from build123d import *

# Parameters (mm, degrees)
SKETCH1_W               = 138
SKETCH1_H               = 63
BOSS_EXTRUDE1_DEPTH     = 2.5
SKETCH3_W               = 28
SKETCH3_H               = 6
CUT_EXTRUDE2_DEPTH      = 10
SKETCH4_W               = 61
SKETCH4_H               = 22
CUT_EXTRUDE3_DEPTH      = 2
SKETCH6_W               = 33
SKETCH6_H               = 19
CUT_EXTRUDE5_DEPTH      = 1.5
SKETCH11_R              = 0.775
CUT_EXTRUDE8_DEPTH      = 6
CUT_EXTRUDE9_DEPTH      = 82.077123777
CUT_EXTRUDE9_DEPTH_BACK = 82.077123777
SKETCH5_R               = 1.575
SKETCH5_R_2             = 1.75
SKETCH16_R              = 6
CUT_EXTRUDE10_DEPTH     = 11
SKETCH19_R              = 1.25
CUT_EXTRUDE12_DEPTH     = 5
SKETCH21_W              = 17
SKETCH21_H              = 2.5
BOSS_EXTRUDE2_DEPTH     = 11
SKETCH22_W              = 63
SKETCH22_H              = 5
BOSS_EXTRUDE3_DEPTH     = 4
SKETCH23_R              = 1.5
BOSS_EXTRUDE4_DEPTH     = 2
FILLET3_R               = 4
FILLET2_R               = 1.5


with BuildPart() as part:
    # Sketch1 → Boss-Extrude1 (new, symmetric)
    with BuildSketch(Plane(origin=(0, 0, 0), x_dir=(1, 0, 0), z_dir=(0, 1, 0))):
        Rectangle(SKETCH1_W, SKETCH1_H)
    extrude(amount=BOSS_EXTRUDE1_DEPTH, both=True)

    # Sketch3 → Cut-Extrude2 (cut)
    with BuildSketch(Plane(origin=(0, 2.5, 0), x_dir=(1, 0, 0), z_dir=(0, 1, 0))):
        with Locations((-36, -14)):
            Rectangle(SKETCH3_W, SKETCH3_H)
        with Locations((36, -14)):
            Rectangle(SKETCH3_W, SKETCH3_H)
        with Locations((36, 14)):
            Rectangle(SKETCH3_W, SKETCH3_H)
        with Locations((-36, 14)):
            Rectangle(SKETCH3_W, SKETCH3_H)
    extrude(amount=-CUT_EXTRUDE2_DEPTH, mode=Mode.SUBTRACT)

    # Sketch4 → Cut-Extrude3 (cut)
    with BuildSketch(Plane(origin=(0, 2.5, 0), x_dir=(1, 0, 0), z_dir=(0, 1, 0))):
        with Locations((-2.5, 0)):
            Rectangle(SKETCH4_W, SKETCH4_H)
    extrude(amount=-CUT_EXTRUDE3_DEPTH, mode=Mode.SUBTRACT)

    # Sketch6 → Cut-Extrude5 (cut)
    with BuildSketch(Plane(origin=(0, 0.5, 0), x_dir=(1, 0, 0), z_dir=(0, 1, 0))):
        with Locations((7.5, 0)):
            Rectangle(SKETCH6_W, SKETCH6_H)
    extrude(amount=-CUT_EXTRUDE5_DEPTH, mode=Mode.SUBTRACT)

    # Sketch11 → Cut-Extrude8 (cut)
    with BuildSketch(Plane(origin=(0, 2.5, 0), x_dir=(1, 0, 0), z_dir=(0, 1, 0))):
        with Locations(Location((-58, 7.62, 0), (0, 0, 270))):
            Circle(SKETCH11_R)
        with Locations(Location((-19.9, 7.62, 0), (0, 0, 270))):
            Circle(SKETCH11_R)
        with Locations(Location((-58, -7.62, 0), (0, 0, 270))):
            Circle(SKETCH11_R)
        with Locations(Location((-19.9, -7.62, 0), (0, 0, 270))):
            Circle(SKETCH11_R)
    extrude(amount=-CUT_EXTRUDE8_DEPTH, mode=Mode.SUBTRACT)

    # Sketch5 → Cut-Extrude9 (cut, two sides: drawn at the far end of the back side and taken through both)
    with BuildSketch(Plane(origin=(0, 0, -11), x_dir=(-1, 0, 0), z_dir=(0, 0, -1)).offset(-CUT_EXTRUDE9_DEPTH_BACK)):
        with Locations((36, 0)):
            Circle(SKETCH5_R)
        with Locations((-36, 0)):
            Circle(SKETCH5_R_2)
    extrude(amount=CUT_EXTRUDE9_DEPTH + CUT_EXTRUDE9_DEPTH_BACK, mode=Mode.SUBTRACT)

    # Sketch16 → Cut-Extrude10 (cut, symmetric)
    with BuildSketch(Plane.XY):
        with Locations((36, 0)):
            Circle(SKETCH16_R)
    extrude(amount=CUT_EXTRUDE10_DEPTH, both=True, mode=Mode.SUBTRACT)

    # Sketch19 → Cut-Extrude12 (cut)
    with BuildSketch(Plane(origin=(0, 2.5, 0), x_dir=(1, 0, 0), z_dir=(0, 1, 0))):
        with Locations(Location((-65.33, 25.32, 0), (0, 0, 270))):
            Circle(SKETCH19_R)
        with Locations(Location((-65.33, -25.32, 0), (0, 0, 90))):
            Circle(SKETCH19_R)
        with Locations(Location((65.33, -25.32, 0), (0, 0, 270))):
            Circle(SKETCH19_R)
        with Locations(Location((65.33, 25.32, 0), (0, 0, 90))):
            Circle(SKETCH19_R)
    extrude(amount=-CUT_EXTRUDE12_DEPTH, mode=Mode.SUBTRACT)

    # Sketch21 → Boss-Extrude2 (add, symmetric)
    with BuildSketch(Plane.XY):
        with Locations((-41.5, 3.75)):
            Rectangle(SKETCH21_W, SKETCH21_H)
    extrude(amount=BOSS_EXTRUDE2_DEPTH, both=True)

    # Sketch22 → Boss-Extrude3 (add)
    with BuildSketch(Plane(origin=(69, 0, 0), x_dir=(0, 0, -1), z_dir=(1, 0, 0))):
        Rectangle(SKETCH22_W, SKETCH22_H)
    boss_extrude3 = extrude(amount=BOSS_EXTRUDE3_DEPTH)

    # Sketch23 → Boss-Extrude4 (add)
    with BuildSketch(Plane(origin=(73, 0, 0), x_dir=(0, 0, -1), z_dir=(1, 0, 0))):
        with Locations((-13, 0)):
            Circle(SKETCH23_R)
        with Locations((13, 0)):
            Circle(SKETCH23_R)
    boss_extrude4 = extrude(amount=BOSS_EXTRUDE4_DEPTH)

    # Mirror1: Boss-Extrude3 across plane
    add(boss_extrude3.mirror(Plane(origin=(0, 0, 0), x_dir=(0, 0, 1), z_dir=(1, 0, 0))))

    # Mirror7: Boss-Extrude4 across plane
    add(boss_extrude4.mirror(Plane(origin=(0, 0, 0), x_dir=(0, 0, 1), z_dir=(1, 0, 0))))

    # Fillet3
    fillet3_edges = [part.edges().sort_by_distance(p)[0] for p in [
        (73, 0, 31.5),
        (73, 0, -31.5),
        (-73, 0, 31.5),
        (-73, 0, -31.5),
    ]]
    fillet(fillet3_edges, radius=FILLET3_R)

    # Fillet2
    fillet2_edges = [part.edges().sort_by_distance(p)[0] for p in [
        (75, 0, 14.5),
        (75, 0, -11.5),
        (-75, 0, 14.5),
        (-75, 0, -11.5),
    ]]
    fillet(fillet2_edges, radius=FILLET2_R)


solid = part.part
The model under review builds one solid part; all positions refer to its coordinate system, in mm. A direction names the side the tool comes from. Round coordinates to 2 decimals unless told otherwise and drop trailing zeros. Write each loop counter-clockwise with the first axis right and the second up, starting at its lowest first coordinate (ties: lowest second). Pieces come first, ordered by that corner, then holes. Notation, with made-up numbers: M 43,-39 L 67,-39 A21 cw 67,-24 Z; hole C 80.25,-38 d8. An arc over 180 degrees is marked long. Use a Markdown table: item, result. Add a question column.
Q1. The part is to be moulded in two halves that separate along Z. For faces 1 (the face through (7, -1, 0)), 2 (the face through (-71.859, 0.035, -30.297)), 3 (the face through (-71.797, 0.035, 30.359)), 4 (the face through (34.383, -0.67, 24.352)), say which applies: pulls with the +Z half, pulls with the -Z half, needs draft (parallel to the pull), parting line crosses it, or undercut.
Q2. To check wall thickness, follow line 1 (X direction, y = -0.25, z = 19.5); line 2 (Z direction, x = 48.5, y = -1.75); line 3 (X direction, y = 0, z = -4) (3 decimals). State the ranges of each line that lie inside material, in increasing order.
Q3. Machinability: for faces 5 (the face through (30, 0, 0)), 6 (the face through (-73.25, 0.07, 14.5)), 7 (the face through (-50, 0, 14)), which of the approach directions +Z, -Z, +X, -X, +Y, -Y give a long, thin tool a straight path to every point of the face, cutting with its end or side? Answer none if there is none.
Q4. We need section A-A, the plane z = -13. State the section outline as (x, y) points, plus the area to 3 significant figures.
Q5. We need section C-C, the plane x = -1. State the section outline as (y, z) points, plus the area to 4 significant figures.
Q6. Insertion check: pin 1 (0.9 mm diameter, centred on x = -58, z = -7.62, fed in from -Y); pin 2 (3 mm diameter, centred on x = 31, z = -11, fed in from +Y); pin 3 (5.5 mm diameter, centred on x = 9.5, z = -3.5, fed in from +Y); pin 4 (1.8 mm diameter, centred on x = -19.9, z = 7.62, fed in from +Y). Each pin has a flat end and moves straight along its axis. Give the tip position at first contact, or say it passes through.
Q7. We need section D-D, the plane y = 3.75. State the section outline as (x, z) points, plus the area to 3 significant figures.
Q8. We need section B-B, the plane x = -46. State the section outline as (y, z) points, plus the area to 3 significant figures.
Findings below:
| question | item | result |
|---|---|---|
| 1 | face 1 | undercut |
| 1 | face 2 | pulls with the -Z half |
| 1 | face 3 | pulls with the +Z half |
| 1 | face 4 | needs draft |
| 2 | line 1 | x = -73 to -37.56, -34.44 to 34.27, 37.73 to 73 |
| 2 | line 2 | z = -31.5 to -17, -11 to 11, 17 to 31.5 |
| 2 | line 3 | x = -73 to -37.575, -34.425 to -9, 24 to 30, 42 to 73 |
| 3 | face 5 | none |
| 3 | face 6 | -X |
| 3 | face 7 | +Y, -Y |
| 4 | outline | M -73.5,-1.5 L -73,-1.5 L -73,-2.5 L -50,-2.5 L -50,2.5 L -73,2.5 L -73,1.5 L -73.5,1.5 A1.5 ccw Z; M -22,-2.5 L 22,-2.5 L 22,2.5 L -22,2.5 Z; M 50,-2.5 L 73,-2.5 L 73,-1.5 L 73.5,-1.5 A1.5 ccw 73.5,1.5 L 73,1.5 L 73,2.5 L 50,2.5 Z |
| 4 | area | 460 mm² |
| 5 | outline | M -2.5,-31.5 L 2.5,-31.5 L 2.5,-11 L 0.5,-11 L 0.5,-9.5 L -1,-9.5 L -1,9.5 L 0.5,9.5 L 0.5,11 L 2.5,11 L 2.5,31.5 L -2.5,31.5 Z |
| 5 | area | 242.5 mm² |
| 6 | pin 1 | passes through |
| 6 | pin 2 | stops at y = 2.5 |
| 6 | pin 3 | stops at y = -1 |
| 6 | pin 4 | stops at y = 0.5 |
| 7 | outline | M -50,-11 L -33,-11 L -33,11 L -50,11 Z |
| 7 | area | 374 mm² |
| 8 | outline | M -2.5,-31.5 L 2.5,-31.5 L 2.5,-17 L -2.5,-17 Z; M -2.5,-11 L 5,-11 L 5,11 L -2.5,11 Z; M -2.5,17 L 2.5,17 L 2.5,31.5 L -2.5,31.5 Z |
| 8 | area | 310 mm² |
